The listing builds one solid part. Answer for the finished solid, in the listing's coordinates (mm). A direction names the side the tool comes from. Coordinates: 2 decimals unless noted, no trailing zeros. Loops run counter-clockwise (first coordinate to the right, second up) from the corner with the lowest first, then second, coordinate; pieces in that order, holes last. Notation, with made-up numbers: M 78.5,34.25 L 89.5,34.25 A33 cw 89.5,71.25 Z; hole C -15,66 d9. An arc over 180 degrees is marked long. Answer as a JSON object with one key per item and string values. Group by question number.
1. Determine the mould class of faces 3 (the face through (6.01, -13.31, 1.52)), 4 (the face through (-1.598, -7, 14)), 5 (the face through (3, 6.613, 2)) for opening direction Y: released by +Y, released by -Y, zero draft, split by the parting line, or undercut.
2. A cutting plane is placed at A-A on x = 15.5. Give the vertices of the cut face in (y, z), and give its area (3 significant figures).
3. A cutting plane is placed at C-C on y = 0.5. Give the vertices of the cut face in (x, z).
4. Given pin 1 (2 mm diameter, centred on x = 16.85, y = -1.94, fed in from +Z); pin 2 (3 mm diameter, centred on x = 20.5, y = -12, fed in from +Z); pin 3 (4 mm diameter, centred on y = -1, z = 15.5, fed in from +X), each flat-ended and moving along its own axis, determine where each tip first touches the part or whether it passes through.
5. A cutting plane is placed at D-D on z = 11. Give the vertices of the cut face in (x, y), and give its area (3 significant figures).
6. Straight lines are drawn through the part: L1, parallel to Z at x = 10, y = 1.25; L2, parallel to X at y = -0.25, z = 3.25; L3, parallel to Y at x = -3.25, z = 18.5. For each, find the intervals that lie inside material, in ascending order.
7. A cutting plane is placed at B-B on z = 2. Give the vertices of the cut face in (x, y), and give its area (3 significant figures).
8. For faces 1 (the face through (-3.119, 4.148, 22.465)), 2 (the face through (12, -7, 3)), determine the directions among +Z, -Z, +X, -X, +Y, -Y from which every point of the face is accessible in a straight line to the end or side of a thin tool.
from build123d import *

# Parameters (mm, degrees)
F0_W     = 9.9
F0_H     = 4.9494949237
F1_DEPTH = 3
F0_W_2   = 3
F0_H_2   = 13.5
F2_DEPTH = 25
F3_D     = 3.5
F3_DEPTH = 12.4
F3_TIP   = 1.0515060833
F5_DEPTH = 30.001
F6_SIZE  = 5


# Not quite as in the source:
# - a feature names something its author has since deleted; it is built from what else it names


with BuildPart() as f1:
    # F0 (on Top) → F1 (new body)
    with BuildSketch(Plane.XY):
        with BuildLine():
            Line((25.4016518593, 6.6133860946), (-1.5983481407, 6.6133860946))
            Line((-1.5983481407, 6.6133860946), (-1.5983481407, -6.8866139054))
            Line((-1.5983481407, -6.8866139054), (4.9016518593, -6.8866139054))
            ThreePointArc((4.9016518593, -6.8866139054), (5.4344267975, -4.2079948582), (6.9516518593, -1.9371189817))
            ThreePointArc((6.9516518593, -1.9371189817), (11.9016518593, 0.1133860946), (16.8516518593, -1.9371189817))
            ThreePointArc((16.8516518593, -1.9371189817), (18.3688769211, -4.2079948582), (18.9016518593, -6.8866139054))
            Line((18.9016518593, -6.8866139054), (25.4016518593, -6.8866139054))
            Line((25.4016518593, -6.8866139054), (25.4016518593, 6.6133860946))
        make_face()
        with BuildLine():
            Line((4.9016518593, -6.8866139054), (-1.5983481407, -6.8866139054))
            Line((-1.5983481407, -6.8866139054), (-1.5983481407, -20.3866139054))
            Line((-1.5983481407, -20.3866139054), (25.4016518593, -20.3866139054))
            Line((25.4016518593, -20.3866139054), (25.4016518593, -6.8866139054))
            Line((25.4016518593, -6.8866139054), (18.9016518593, -6.8866139054))
            ThreePointArc((18.9016518593, -6.8866139054), (18.3688769211, -9.5652329526), (16.8516518593, -11.8361088292))
            ThreePointArc((16.8516518593, -11.8361088292), (11.9016518593, -13.8866139054), (6.9516518593, -11.8361088292))
            ThreePointArc((6.9516518593, -11.8361088292), (5.4344267975, -9.5652329526), (4.9016518593, -6.8866139054))
        make_face()
        with BuildLine():
            ThreePointArc((16.8516518593, -1.9371189817), (11.9016518593, 0.1133860946), (6.9516518593, -1.9371189817))
            Line((6.9516518593, -1.9371189817), (16.8516518593, -1.9371189817))
        make_face()
        with BuildLine():
            ThreePointArc((6.9516518593, -1.9371189817), (5.4344267975, -4.2079948582), (4.9016518593, -6.8866139054))
            Line((4.9016518593, -6.8866139054), (6.9516518593, -6.8866139054))
            Line((6.9516518593, -6.8866139054), (6.9516518593, -1.9371189817))
        make_face()
        with Locations((11.9016518593, -4.4118664436)):
            Rectangle(F0_W, F0_H)
        with BuildLine():
            Line((16.8516518593, -6.8866139054), (18.9016518593, -6.8866139054))
            ThreePointArc((18.9016518593, -6.8866139054), (18.3688769211, -4.2079948582), (16.8516518593, -1.9371189817))
            Line((16.8516518593, -1.9371189817), (16.8516518593, -6.8866139054))
        make_face()
        with BuildLine():
            ThreePointArc((16.8516518593, -11.8361088292), (18.3688769211, -9.5652329526), (18.9016518593, -6.8866139054))
            Line((18.9016518593, -6.8866139054), (16.8516518593, -6.8866139054))
            Line((16.8516518593, -6.8866139054), (16.8516518593, -11.8361088292))
        make_face()
        with Locations((11.9016518593, -9.3613613673)):
            Rectangle(F0_W, F0_H)
        with BuildLine():
            Line((6.9516518593, -6.8866139054), (4.9016518593, -6.8866139054))
            ThreePointArc((4.9016518593, -6.8866139054), (5.4344267975, -9.5652329526), (6.9516518593, -11.8361088292))
            Line((6.9516518593, -11.8361088292), (6.9516518593, -6.8866139054))
        make_face()
        with BuildLine():
            Line((16.8516518593, -11.8361088292), (6.9516518593, -11.8361088292))
            ThreePointArc((6.9516518593, -11.8361088292), (11.9016518593, -13.8866139054), (16.8516518593, -11.8361088292))
        make_face()
    extrude(amount=F1_DEPTH)

    # F0 (on Top) → F2 (join)
    with BuildSketch(Plane.XY):
        with Locations((-3.0983481407, -0.1366139054)):
            Rectangle(F0_W_2, F0_H_2)
        with Locations((-3.0983481407, -13.6366139054)):
            Rectangle(F0_W_2, F0_H_2)
    extrude(amount=F2_DEPTH)

    # F3
    with Locations(Plane(origin=(0, 0, 0), x_dir=(1, 0, 0), z_dir=(0, 0, -1))):
        with Locations((16.8516518593, 1.9371189817), (6.9516518593, 11.8361088292)):
            Hole(F3_D / 2, depth=F3_DEPTH)
            with Locations((0, 0, -(F3_DEPTH + F3_TIP / 2))):  # 118° drill point
                Cone(0, F3_D / 2, F3_TIP, mode=Mode.SUBTRACT)

    # F4 (on face) → F5 (cut, through all)
    with BuildSketch(Plane(origin=(-4.5983481407, 0, 0), x_dir=(0, -1, 0), z_dir=(-1, 0, 0))):
        Polygon((20.3866139054, 25), (15.3866139054, 25), (20.3866139054, 15), align=None)
    extrude(amount=-F5_DEPTH, mode=Mode.SUBTRACT)

    # F6
    f6_edges = [f1.edges().sort_by_distance(p)[0] for p in [
        (25.401652, -20.386614, 1.5),
        (25.401652, 6.613386, 1.5),
        (-3.098348, 6.613386, 25),
    ]]
    chamfer(f6_edges, length=F6_SIZE)


solid = f1.part
From the geometry:
{
 "1": {"face 3": "undercut", "face 4": "zero draft", "face 5": "released by +Y"},
 "2": {"outline": "M -20.39,0 L -3.05,0 L -3.05,3 L -20.39,3 Z; M -0.83,0 L 6.61,0 L 6.61,3 L -0.83,3 Z", "area": "74.3 mm²"},
 "3": {"outline": "M -4.6,0 L 25.4,0 L 25.4,3 L -1.6,3 L -1.6,25 L -4.6,25 Z"},
 "4": {"pin 1": "passes through", "pin 2": "stops at z = 3", "pin 3": "stops at x = -1.6"},
 "5": {"outline": "M -4.6,-20.39 L -1.6,-20.39 L -1.6,6.61 L -4.6,6.61 Z", "area": "81.0 mm²"},
 "6": {"L1": "z = 0 to 3", "L2": "x = -4.6 to -1.6", "L3": "y = -18.64 to 6.61"},
 "7": {"outline": "M -4.6,-20.39 L 20.4,-20.39 L 25.4,-15.39 L 25.4,1.61 L 20.4,6.61 L -4.6,6.61 Z; hole C 6.95,-11.84 d3.5; hole C 16.85,-1.94 d3.5", "area": "766 mm²"},
 "8": {"face 1": "+Z, +X, -X, +Y", "face 2": "+Z, +X, +Y, -Y"}
}
